Design review of the part built by this model. Coordinates are the model's own, in mm. Face numbers are marked on the shaded views. Round coordinates to 2 decimals unless told otherwise and drop trailing zeros. Order: outer loops, then holes, each group sorted by start corner. A loop starts at its lowest first (then second) coordinate and runs counter-clockwise, first axis right, second up. Notation, with made-up numbers: (-9, 56.25) - (10, 56.25) arc R3 cw to (10, 60.25) - close; hole circle Ø1 at (26, 32). An arc over 180 degrees is marked (long way). Use CSV: the item, a comma, the result in double quotes.
from build123d import *

# Parameters (mm, degrees)
F0_R      = 27
F1_DEPTH  = 6
F2_R      = 26
F3_DEPTH  = 10
F4_R      = 27
F5_DEPTH  = 19
F6_R      = 26
F7_DEPTH  = 10
F8_R      = 27
F9_DEPTH  = 6
F10_R     = 22.6
F11_DEPTH = 51.001


with BuildPart() as f1:
    # F0 (on Top) → F1 (new body)
    with BuildSketch(Plane.XY):
        Circle(F0_R)
    extrude(amount=F1_DEPTH)

    # F2 (on face) → F3 (join)
    with BuildSketch(Plane.XY.offset(6)):
        Circle(F2_R)
    extrude(amount=F3_DEPTH)

    # F4 (on face) → F5 (join)
    with BuildSketch(Plane.XY.offset(16)):
        Circle(F4_R)
    extrude(amount=F5_DEPTH)

    # F6 (on face) → F7 (join)
    with BuildSketch(Plane.XY.offset(35)):
        Circle(F6_R)
    extrude(amount=F7_DEPTH)

    # F8 (on face) → F9 (join)
    with BuildSketch(Plane.XY.offset(45)):
        Circle(F8_R)
    extrude(amount=F9_DEPTH)

    # F10 (on face) → F11 (cut, through all)
    with BuildSketch(Plane(origin=(0, 0, 0), x_dir=(1, 0, 0), z_dir=(0, 0, -1))):
        Circle(F10_R)
    extrude(amount=-F11_DEPTH, mode=Mode.SUBTRACT)


solid = f1.part
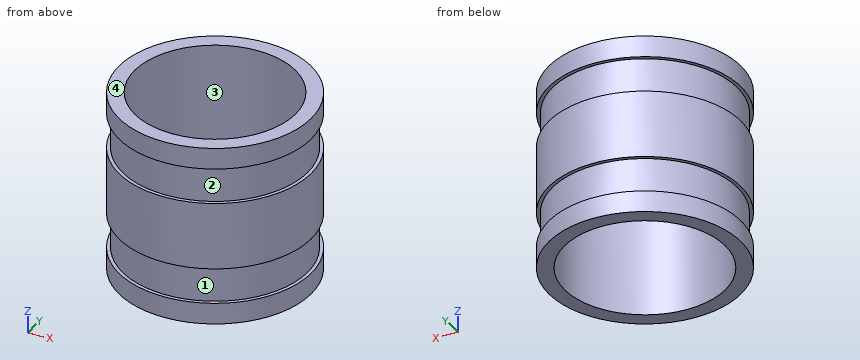
1) We need section D-D (z = 36.5). Give the boundary of the cut face in (x, y).
Data:
outline,"circle Ø52 at (0, 0); hole circle Ø45.2 at (0, 0)"
2) The part is to be moulded in two halves that separate along Z. For the marked faces 1, 2, 3 and 4, say which applies: +Z half, -Z half, draft (parallel to the pull), parting line (faces both ways), or undercut.
Data:
face 1,"undercut"
face 2,"undercut"
face 3,"draft"
face 4,"+Z half"
3) Insertion check: pin 1 Ø4 at (y, z) = (11.5, 18.5) entering from +X; pin 2 Ø4 at (x, z) = (8, 10) entering from +Y; pin 3 Ø2 at (y, z) = (-18.5, 10) entering from -X. Each pin has a flat end and moves straight along its axis. Give the tip position at first contact, or say it passes through.
Data:
pin 1,"stops at x = 25.27"
pin 2,"stops at y = 25.3"
pin 3,"stops at x = -19.23"
4) We need section C-C (z = 47.5). Give the boundary of the cut face in (x, y).
Data:
outline,"circle Ø54 at (0, 0); hole circle Ø45.2 at (0, 0)"
5) To check wall thickness, follow L1, parallel to Z at x = -12.5, y = 23; L2, parallel to Y at x = 0, z = 40; L3, parallel to Y at x = 0, z = 21.5. State the ranges of each line that lie inside material, in increasing order. Write a range as from..to.
Data:
L1,"z = 0..6, 16..35, 45..51"
L2,"y = -26..-22.6, 22.6..26"
L3,"y = -27..-22.6, 22.6..27"
6) We need section A-A (x = 0). Give the boundary of the cut face in (y, z), then the cut area to 3 significant figures.
Data:
outline,"(-27, 0) - (-22.6, 0) - (-22.6, 51) - (-27, 51) - (-27, 45) - (-26, 45) - (-26, 35) - (-27, 35) - (-27, 16) - (-26, 16) - (-26, 6) - (-27, 6) - close; (22.6, 0) - (27, 0) - (27, 6) - (26, 6) - (26, 16) - (27, 16) - (27, 35) - (26, 35) - (26, 45) - (27, 45) - (27, 51) - (22.6, 51) - close"
area,"409 mm2"
